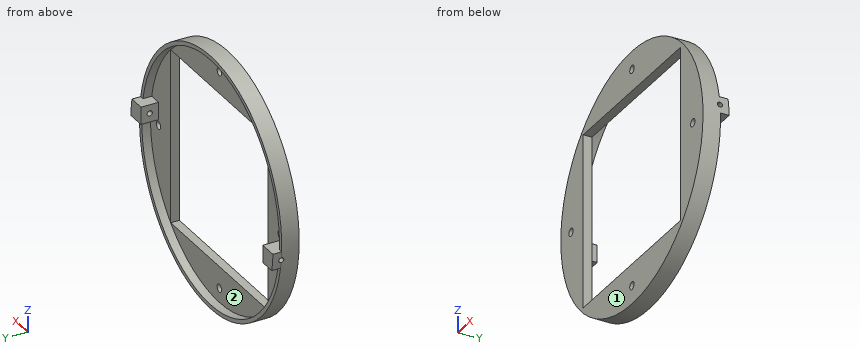
from build123d import *
from build123d.topology import SkipClean

# Parameters (mm, degrees)
SKETCH1_R           = 76
SKETCH1_W           = 100
SKETCH1_H           = 100
BOSS_EXTRUDE1_DEPTH = 5
SKETCH2_R           = 2.25
CUT_EXTRUDE1_DEPTH  = 10
SKETCH3_R           = 73
SKETCH3_R_2         = 70.710678119
BOSS_EXTRUDE2_DEPTH = 5
CUT_EXTRUDE2_START  = -5
SKETCH4_R           = 76
SKETCH4_R_2         = 73
CUT_EXTRUDE2_DEPTH  = 5
BOSS_EXTRUDE4_DEPTH = 10
CUT_EXTRUDE3_DEPTH  = 23
CUT_EXTRUDE4_DEPTH  = 21


with BuildPart() as part:
    # Sketch1 → Boss-Extrude1 (new body)
    with BuildSketch(Plane(origin=(0, 0, 0), x_dir=(1, 0, 0), z_dir=(0, 1, 0))):
        with Locations(Location((0, 0, 0), (0, 0, 270))):
            Circle(SKETCH1_R)
        Rectangle(SKETCH1_W, SKETCH1_H, mode=Mode.SUBTRACT)
    extrude(amount=BOSS_EXTRUDE1_DEPTH)

    # Sketch2 → Cut-Extrude1 (cut)
    with BuildSketch(Plane(origin=(0, 5, 0), x_dir=(1, 0, 0), z_dir=(0, 1, 0))):
        with Locations(Location((-62.5, 0, 0), (0, 0, 270))):
            Circle(SKETCH2_R)
        with Locations(Location((0, 62.5, 0), (0, 0, 270))):
            Circle(SKETCH2_R)
        with Locations(Location((62.5, 0, 0), (0, 0, 270))):
            Circle(SKETCH2_R)
        with Locations(Location((0, -62.5, 0), (0, 0, 270))):
            Circle(SKETCH2_R)
    extrude(amount=-CUT_EXTRUDE1_DEPTH, mode=Mode.SUBTRACT)

    # Sketch3 → Boss-Extrude2 (add)
    with BuildSketch(Plane(origin=(0, 5, 0), x_dir=(1, 0, 0), z_dir=(0, 1, 0))):
        with Locations(Location((0, 0, 0), (0, 0, 270))):
            Circle(SKETCH3_R)
        with Locations(Location((0, 0, 0), (0, 0, 135))):
            Circle(SKETCH3_R_2, mode=Mode.SUBTRACT)
    extrude(amount=BOSS_EXTRUDE2_DEPTH)

    # Sketch4 → Cut-Extrude2 (cut)
    with BuildSketch(Plane(origin=(0, 5, 0), x_dir=(1, 0, 0), z_dir=(0, 1, 0)).offset(CUT_EXTRUDE2_START)):
        Circle(SKETCH4_R)
        with Locations(Location((0, 0, 0), (0, 0, 270))):
            Circle(SKETCH4_R_2, mode=Mode.SUBTRACT)
    extrude(amount=CUT_EXTRUDE2_DEPTH, mode=Mode.SUBTRACT)

    # Sketch7 → Boss-Extrude4 (add)
    with SkipClean():  # the faces are left unmerged after this step: merging them gives an invalid solid
        with BuildSketch(Plane(origin=(0, 5, 0), x_dir=(1, 0, 0), z_dir=(0, 1, 0))):
            with BuildLine():
                ThreePointArc((-71.787446674, 13.25), (-72.530079982, 8.269673379), (-72.927618225, 3.25))
                Line((-72.927618225, 3.25), (-62.5, 3.25))
                Line((-62.5, 3.25), (-62.5, 13.25))
                Line((-62.5, 13.25), (-71.787446674, 13.25))
            make_face()
            with BuildLine():
                Line((72.927618225, -3.25), (62.5, -3.25))
                Line((62.5, -3.25), (62.5, -13.25))
                Line((62.5, -13.25), (71.787446674, -13.25))
                ThreePointArc((71.787446674, -13.25), (72.530079982, -8.269673379), (72.927618225, -3.25))
            make_face()
        extrude(amount=BOSS_EXTRUDE4_DEPTH)

    # Sketch8 → Cut-Extrude3 (cut)
    with SkipClean():  # the faces are left unmerged after this step: merging them gives an invalid solid
        with BuildSketch(Plane.ZY.offset(-62.5)):
            with BuildLine():
                ThreePointArc((9.75, 10), (9.310660172, 11.060660172), (8.25, 11.5))
                Line((8.25, 11.5), (8.25, 8.5))
                ThreePointArc((8.25, 8.5), (9.310660172, 8.939339828), (9.75, 10))
            make_face()
            with BuildLine():
                Line((8.25, 8.5), (8.25, 11.5))
                ThreePointArc((8.25, 11.5), (6.75, 10), (8.25, 8.5))
            make_face()
        extrude(amount=-CUT_EXTRUDE3_DEPTH, mode=Mode.SUBTRACT)

    # Sketch9 → Cut-Extrude4 (cut)
    with BuildSketch(Plane(origin=(-62.5, 0, 0), x_dir=(0, 0, -1), z_dir=(1, 0, 0))):
        with BuildLine():
            ThreePointArc((9.75, 10), (9.310660172, 11.060660172), (8.25, 11.5))
            Line((8.25, 11.5), (8.25, 8.5))
            ThreePointArc((8.25, 8.5), (9.310660172, 8.939339828), (9.75, 10))
        make_face()
        with BuildLine():
            Line((8.25, 8.5), (8.25, 11.5))
            ThreePointArc((8.25, 11.5), (6.75, 10), (8.25, 8.5))
        make_face()
    extrude(amount=-CUT_EXTRUDE4_DEPTH, mode=Mode.SUBTRACT)


solid = part.part
Design review of the part built by this model. Coordinates are the model's own, in mm. Face numbers are marked on the shaded views. Round coordinates to 2 decimals unless told otherwise and drop trailing zeros. Loops run counter-clockwise (first coordinate to the right, second up) from the corner with the lowest first, then second, coordinate; pieces in that order, holes last. Notation, with made-up numbers: (1.5, 77) -> (28.5, 77) arc R30 cw to (28.5, 110) -> close; hole circle Ø9 at (10, 32). An arc over 180 degrees is marked (long way). Use one line per item in the form item = value. Start each with the question number.
Q1. For pin 1 Ø5.5 at (y, z) = (2, -8) entering from -X; pin 2 Ø4 at (x, y) = (-11, 2.5) entering from -Z; pin 3 Ø7 at (x, z) = (62.5, 0) entering from -Y; pin 4 Ø5 at (x, y) = (-18, 9) entering from +Z, all flat-tipped, find the tip position at first contact; note any pin that passes through.
Q2. We need section A-A on x = 0. Give the boundary of the cut face in (y, z), then the cut area to 3 significant figures.
Q3. We need section B-B on z = -34. Give the boundary of the cut face in (x, y).
Q4. Wall thickness on line 1 along X through (y, z) = (3.65, 0); line 2 along Z through (x, y) = (-1.5, 6.25); line 3 along Z through (x, y) = (7, 4.5): over which ranges is each line inside the solid? List them lowest first. Write a range as [from, to].
Q5. We need section D-D on x = 28. Give the boundary of the cut face in (y, z), then the cut area to 3 significant figures.
Q6. Draft analysis for pull direction X (two halves, no side actions). For the marked faces 1 and 2, state which applies: +X half, -X half, draft (parallel to the pull), parting line (faces both ways), or undercut.
Calculated:
q1.pin_1 = -72.81
q1.pin_2 = -72.44
q1.pin_3 = 0
q1.pin_4 = 71.34
q2.outline = (0, -73) -> (10, -73) -> (10, -70.71) -> (5, -70.71) -> (5, -64.75) -> (0, -64.75) -> close; (0, -60.25) -> (5, -60.25) -> (5, -50) -> (0, -50) -> close; (0, 50) -> (5, 50) -> (5, 60.25) -> (0, 60.25) -> close; (0, 64.75) -> (5, 64.75) -> (5, 70.71) -> (10, 70.71) -> (10, 73) -> (0, 73) -> close
q2.area = 208 mm²
q3.outline = (-64.6, 0) -> (-50, 0) -> (-50, 5) -> (-62, 5) -> (-62, 10) -> (-64.6, 10) -> close; (50, 0) -> (64.6, 0) -> (64.6, 10) -> (62, 10) -> (62, 5) -> (50, 5) -> close
q4.line_1 = [-73, -64.75], [-60.25, -50], [50, 60.25], [64.75, 73]
q4.line_2 = [-72.98, -70.69], [70.69, 72.98]
q4.line_3 = [-72.66, -50], [50, 72.66]
q5.outline = (0, -67.42) -> (10, -67.42) -> (10, -64.93) -> (5, -64.93) -> (5, -50) -> (0, -50) -> close; (0, 50) -> (5, 50) -> (5, 64.93) -> (10, 64.93) -> (10, 67.42) -> (0, 67.42) -> close
q5.area = 199 mm²
q6.face_1 = draft
q6.face_2 = undercut
